Could you check a few things on this model? Use its own coordinates, in mm. Coordinates: 2 decimals unless noted, no trailing zeros. Write each loop counter-clockwise with the first axis right and the second up, starting at its lowest first coordinate (ties: lowest second). Pieces come first, ordered by that corner, then holes.
Item 1: I want a section at B-B on x = 26.5. Please give me the cut outline in (y, z), then the cut area to 3 significant figures.
Item 2: For P1, Ø6, axis at y = 1, z = 1, coming from the +X side; P2, Ø5, axis at x = -21.5, z = -8, coming from the -Y side; P3, Ø1, axis at x = -1.5, z = -6.5, coming from the +Y side; P4, Ø5, axis at x = -24.5, y = 5.5, coming from the +Z side, each with a flat end and sliding along its axis, tell me the tip position at first contact or that it passes through.
Item 3: I want a section at A-A on y = -8.5. Please give me the cut outline in (x, z).
Item 4: If I drill on probe 1 along X at (y, z) = (-2.25, -8.5); probe 2 along Y at (x, z) = (-10, 0); probe 3 along Z at (x, y) = (-40, -0.25), over which ranges is the centre line in solid material (lowest first)?
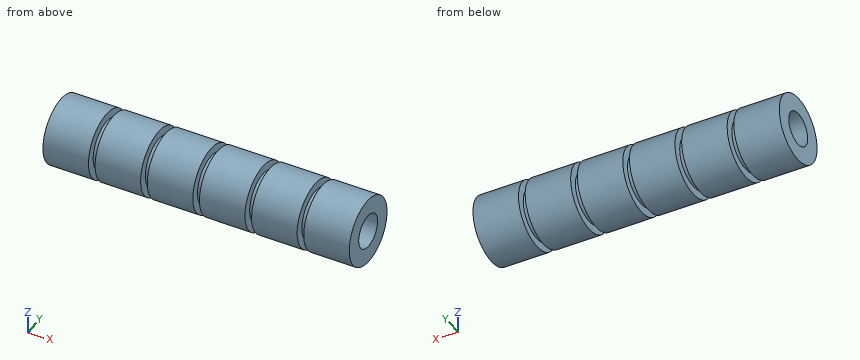
from build123d import *

# Parameters (mm, degrees)
SKETCH_1_R      = 8.5
SKETCH_1_R_2    = 5
EXTRUDE_1_DEPTH = 46
SKETCH_3_W      = 2
SKETCH_3_H      = 1
SKETCH_4_W      = 13.666666667
SKETCH_4_H      = 1.5
SKETCH_4_W_2    = 13.666666666


with BuildPart() as part:
    # 草圖1 → 填料-伸長1 (new body, symmetric)
    with BuildSketch(Plane(origin=(0, 0, 0), x_dir=(0, 0, -1), z_dir=(1, 0, 0))):
        Circle(SKETCH_1_R)
        Circle(SKETCH_1_R_2, mode=Mode.SUBTRACT)
    extrude(amount=EXTRUDE_1_DEPTH, both=True)

    # 草圖3 → 除料-旋轉1 (revolve, cut)
    with BuildSketch(Plane.XY):
        with Locations((31.333333333, 8)):
            Rectangle(SKETCH_3_W, SKETCH_3_H)
        with Locations((15.666666667, 8)):
            Rectangle(SKETCH_3_W, SKETCH_3_H)
        with Locations((0, 8)):
            Rectangle(SKETCH_3_W, SKETCH_3_H)
        with Locations((-15.666666667, 8)):
            Rectangle(SKETCH_3_W, SKETCH_3_H)
        with Locations((-31.333333333, 8)):
            Rectangle(SKETCH_3_W, SKETCH_3_H)
    revolve(axis=Axis((-98.82156335, 0, 0), (1, 0, 0)), mode=Mode.SUBTRACT)

    # 草圖4 → 旋轉2 (revolve)
    with BuildSketch(Plane.XY):
        with Locations((-39.166666666, 9.25)):
            Rectangle(SKETCH_4_W, SKETCH_4_H)
        with Locations((-23.5, 9.25)):
            Rectangle(SKETCH_4_W_2, SKETCH_4_H)
        with Locations((-7.833333334, 9.25)):
            Rectangle(SKETCH_4_W, SKETCH_4_H)
        with Locations((7.833333334, 9.25)):
            Rectangle(SKETCH_4_W, SKETCH_4_H)
        with Locations((23.5, 9.25)):
            Rectangle(SKETCH_4_W_2, SKETCH_4_H)
        with Locations((39.166666666, 9.25)):
            Rectangle(SKETCH_4_W, SKETCH_4_H)
    revolve(axis=Axis((58.089826766, 0, 0), (-1, 0, 0)))


solid = part.part
Response values:
1. outline: circle Ø20 at (0, 0); hole circle Ø10 at (0, 0)
1. area: 236 mm2
2. P1: passes through
2. P2: stops at y = -8.35
2. P3: stops at y = 8
2. P4: stops at z = 9.54
3. outline: (-46, -5.27) - (-32.33, -5.27) - (-32.33, 5.27) - (-46, 5.27) - close; (-30.33, -5.27) - (-16.67, -5.27) - (-16.67, 5.27) - (-30.33, 5.27) - close; (-14.67, -5.27) - (-1, -5.27) - (-1, 5.27) - (-14.67, 5.27) - close; (1, -5.27) - (14.67, -5.27) - (14.67, 5.27) - (1, 5.27) - close; (16.67, -5.27) - (30.33, -5.27) - (30.33, 5.27) - (16.67, 5.27) - close; (32.33, -5.27) - (46, -5.27) - (46, 5.27) - (32.33, 5.27) - close
4. probe 1: x = -46 to -32.33, -30.33 to -16.67, -14.67 to -1, 1 to 14.67, 16.67 to 30.33, 32.33 to 46
4. probe 2: y = -10 to -5, 5 to 10
4. probe 3: z = -10 to -4.99, 4.99 to 10
